from build123d import *

# Parameters (mm, degrees)
SKETCH1_W           = 66
SKETCH1_H           = 44
BOSS_EXTRUDE1_DEPTH = 12
CHAMFER1_SIZE       = 12
SKETCH2_W           = 44
SKETCH2_H           = 48
BOSS_EXTRUDE2_DEPTH = 12
FILLET1_RADIUS      = 22
FILLET1_LENGTH      = 12
BOSS_EXTRUDE3_DEPTH = 6


with BuildPart() as part:
    # Sketch1 → Boss-Extrude1 (new body)
    with BuildSketch(Plane(origin=(0, 0, 0), x_dir=(1, 0, 0), z_dir=(0, 1, 0))):
        Rectangle(SKETCH1_W, SKETCH1_H)
    extrude(amount=BOSS_EXTRUDE1_DEPTH)

    # Chamfer1
    chamfer1_edges = [part.edges().sort_by_distance(p)[0] for p in [
        (33, 6, 22),
        (33, 6, -22),
    ]]
    chamfer(chamfer1_edges, length=CHAMFER1_SIZE)

    # Sketch2 → Boss-Extrude2 (add)
    with BuildSketch(Plane.ZY.offset(33)):
        with Locations((0, 36)):
            Rectangle(SKETCH2_W, SKETCH2_H)
    extrude(amount=-BOSS_EXTRUDE2_DEPTH)

    # Fillet1: full round fillet: the end face becomes a half cylinder, R = half its width
    fillet1_face = Plane((-27, 60, 0), x_dir=(-1, 0, 0), z_dir=(0, 1, 0))  # on the end face: x along it, z out of the body
    fillet1_slab = fillet1_face.offset(-FILLET1_RADIUS / 2) * Box(FILLET1_LENGTH, 2 * FILLET1_RADIUS, FILLET1_RADIUS, mode=Mode.PRIVATE)  # the body's end, R deep
    fillet1_round = Plane((-27, 38, 0), x_dir=(0, 1, 0), z_dir=(-1, 0, 0)) * Cylinder(FILLET1_RADIUS, FILLET1_LENGTH, mode=Mode.PRIVATE)  # its axis R under the face
    add(fillet1_slab - fillet1_round, mode=Mode.SUBTRACT)

    # Sketch4 → Boss-Extrude3 (add, symmetric)
    with BuildSketch(Plane.XY):
        Polygon((-21, 54), (33, 12), (-21, 12), align=None)
    extrude(amount=BOSS_EXTRUDE3_DEPTH, both=True)


solid = part.part
Check sheet for the modelled part. Datum: model origin and axes. Units: mm. A direction names the side the tool comes from. Give positions to 0.01 mm unless a question says otherwise; leave off trailing zeros. Loops run counter-clockwise (first coordinate to the right, second up) from the corner with the lowest first, then second, coordinate; pieces in that order, holes last. Notation, with made-up numbers: M 62,-14.5 L 109,-14.5 A31 cw 109,11.5 Z; hole C 22,47.25 d8. An arc over 180 degrees is marked long. Use a Markdown table: item, result. Add a question column.
Q1. Sectioned sample at C-C, the plane y = 8.5. Record the cut outline in (x, z).
Q2. Scan lines: line 1 along X through (y, z) = (28.5, 18); line 2 along Y through (x, z) = (7.5, 10); line 3 along Z through (x, y) = (-15.5, 15). Record each from-to range of solid material in increasing order. Write a range as [from, to].
Q3. Go/stop test with flat-tipped pins: pin 1 (8 mm diameter, centred on x = 1.5, z = 5, fed in from -Y); pin 2 (8 mm diameter, centred on y = 25, z = 12.5, fed in from +X); pin 3 (1.5 mm diameter, centred on y = 23.5, z = -4.5, fed in from +X); pin 4 (6 mm diameter, centred on x = -14, y = 40.5, fed in from +Z). Record where each tip stops, or that it passes through.
Q4. Tool access check on faces 1 (the flat face through (27, 6, 16)), 2 (the flat face through (-6, 24, 6)), 3 (the flat face through (6, 12, -14)), 4 (the flat face through (33, 6, 0)), 5 (the flat face through (-21, 36, 9)). Record the directions out of +Z, -Z, +X, -X, +Y, -Y that give a thin tool (end or side, any length) a straight path to the whole face; none if there is none.
Q5. Sectioned sample at A-A, the plane x = 19.5. Record the cut outline in (y, z), then the cut area to 3 significant figures.
Q6. Sectioned sample at D-D, the plane x = -7. Record the cut outline in (y, z).
Q7. Sectioned sample at B-B, the plane z = 0. Record the cut outline in (x, y).
Verdict:
| question | item | result |
|---|---|---|
| 1 | outline | M -33,-22 L 21,-22 L 33,-10 L 33,10 L 21,22 L -33,22 Z |
| 2 | line 1 | [-33, -21] |
| 2 | line 2 | [0, 12] |
| 2 | line 3 | [-6, 6] |
| 3 | pin 1 | y = 0 |
| 3 | pin 2 | x = -21 |
| 3 | pin 3 | x = 19.18 |
| 3 | pin 4 | z = 6 |
| 4 | face 1 | +Z, +X, +Y, -Y |
| 4 | face 2 | +Z, +X, +Y |
| 4 | face 3 | -Z, +X, +Y |
| 4 | face 4 | +Z, -Z, +X, +Y, -Y |
| 4 | face 5 | +X, +Y |
| 5 | outline | M 0,-22 L 12,-22 L 12,-6 L 22.5,-6 L 22.5,6 L 12,6 L 12,22 L 0,22 Z |
| 5 | area | 654 mm^2 |
| 6 | outline | M 0,-22 L 12,-22 L 12,-6 L 43.11,-6 L 43.11,6 L 12,6 L 12,22 L 0,22 Z |
| 7 | outline | M -33,0 L 33,0 L 33,12 L -21,54 L -21,60 L -33,60 Z |
